```python
from build123d import *

# Parameters (mm, degrees)
SKETCH1_W           = 70
SKETCH1_H           = 70
SKETCH1_R           = 1.625
BOSS_EXTRUDE1_DEPTH = 4
SKETCH2_W           = 2.725639952
SKETCH2_H           = 70
CUT_EXTRUDE1_DEPTH  = 2
CHAMFER1_SIZE       = 1


with BuildPart() as part:
    # Sketch1 → Boss-Extrude1 (new body)
    with BuildSketch(Plane.XY):
        with Locations((35, 35)):
            Rectangle(SKETCH1_W, SKETCH1_H)
        with Locations((4.5, 65.5)):
            Circle(SKETCH1_R, mode=Mode.SUBTRACT)
        with Locations((65.5, 65.5)):
            Circle(SKETCH1_R, mode=Mode.SUBTRACT)
        with Locations((65.5, 4.5)):
            Circle(SKETCH1_R, mode=Mode.SUBTRACT)
        with Locations((4.5, 4.5)):
            Circle(SKETCH1_R, mode=Mode.SUBTRACT)
    extrude(amount=BOSS_EXTRUDE1_DEPTH)

    # Sketch2 → Cut-Extrude1 (cut)
    with BuildSketch(Plane.XY.offset(4)):
        with Locations((11.296666841, 35)):
            Rectangle(SKETCH2_W, SKETCH2_H)
        with Locations((16.496666841, 35)):
            Rectangle(SKETCH2_W, SKETCH2_H)
        with Locations((21.696666841, 35)):
            Rectangle(SKETCH2_W, SKETCH2_H)
        with Locations((26.896666841, 35)):
            Rectangle(SKETCH2_W, SKETCH2_H)
        with Locations((32.096666841, 35)):
            Rectangle(SKETCH2_W, SKETCH2_H)
        with Locations((37.296666841, 35)):
            Rectangle(SKETCH2_W, SKETCH2_H)
        with Locations((42.496666841, 35)):
            Rectangle(SKETCH2_W, SKETCH2_H)
        with Locations((47.696666841, 35)):
            Rectangle(SKETCH2_W, SKETCH2_H)
        with Locations((52.896666841, 35)):
            Rectangle(SKETCH2_W, SKETCH2_H)
        with Locations((58.096666841, 35)):
            Rectangle(SKETCH2_W, SKETCH2_H)
    extrude(amount=-CUT_EXTRUDE1_DEPTH, mode=Mode.SUBTRACT)

    # Chamfer1
    chamfer1_edges = [part.edges().sort_by_distance(p)[0] for p in [
        (70, 35, 4),
        (64.729743409, 70, 4),
        (55.496666841, 70, 4),
        (50.296666841, 70, 4),
        (45.096666841, 70, 4),
        (39.896666841, 70, 4),
        (34.696666841, 70, 4),
        (29.496666841, 70, 4),
        (24.296666841, 70, 4),
        (19.096666841, 70, 4),
        (13.896666841, 70, 4),
        (4.966923432, 70, 4),
        (0, 35, 4),
        (13.896666841, 0, 4),
        (19.096666841, 0, 4),
        (24.296666841, 0, 4),
        (29.496666841, 0, 4),
        (34.696666841, 0, 4),
        (39.896666841, 0, 4),
        (45.096666841, 0, 4),
        (50.296666841, 0, 4),
        (55.496666841, 0, 4),
        (64.729743409, 0, 4),
        (4.966923432, 0, 4),
    ]]
    chamfer(chamfer1_edges, length=CHAMFER1_SIZE)


solid = part.part
```
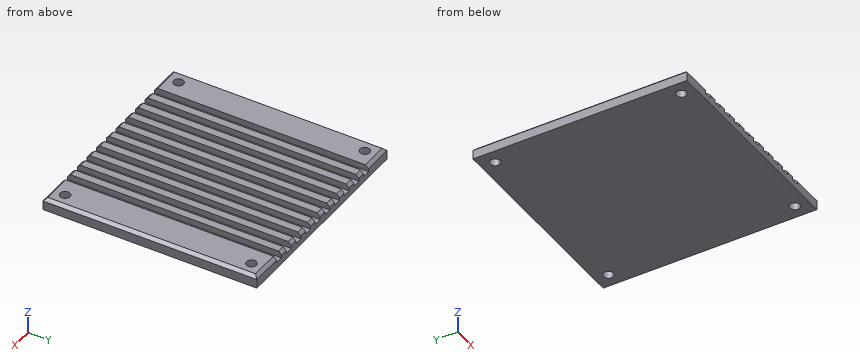
Geometry check sheet. Reference: the model listing, model coordinates, mm. Coordinates: 2 decimals unless noted, no trailing zeros. Order: outer loops, then holes, each group sorted by start corner. A loop starts at its lowest first (then second) coordinate and runs counter-clockwise, first axis right, second up.
Item 1: Depth check by flat-ended pin: pin 1 (8 mm diameter, centred on x = 60.5, y = 40.5, fed in from -Z); pin 2 (2 mm diameter, centred on x = 32, y = 25.5, fed in from +Z); pin 3 (3 mm diameter, centred on x = 65.5, y = 65.5, fed in from -Z). Enter the tip coordinate at first touch or a pass-through.
Item 2: Section check A-A (x = 65.5). Enter the section's corners in (y, z) (3 decimals).
Item 3: Scan lines: line 1 along Y through (x, z) = (4.5, 0.95) (3 decimals); line 2 along Y through (x, z) = (5.5, 0.9). Record each from-to range of solid material in increasing order.
Item 4: Section check B-B (y = 65.5). Count the separate pieces of the cut face and the enclosed holes in it, plus the area to 3 significant figures.
Check sheet entries:
1. pin 1: stops at z = 0
1. pin 2: stops at z = 2
1. pin 3: passes through
2. outline: (0, 0) - (2.875, 0) - (2.875, 4) - (1, 4) - (0, 3) - close; (6.125, 0) - (63.875, 0) - (63.875, 4) - (6.125, 4) - close; (67.125, 0) - (70, 0) - (70, 3) - (69, 4) - (67.125, 4) - close
3. line 1: y = 0 to 2.875, 6.125 to 63.875, 67.125 to 70
3. line 2: y = 0 to 3.22, 5.78 to 64.22, 66.78 to 70
4. separate pieces: 3
4. enclosed holes: 0
4. area: 198 mm2
